For this review, take the finished solid that the model builds, in its own axes (mm). A direction names the side the tool comes from. Coordinates: 2 decimals unless noted, no trailing zeros. Use one line per item in the form item = value.
```python
from build123d import *

# Parameters (mm, degrees)
F0_W     = 400
F0_H     = 50
F1_DEPTH = 300
F3_DEPTH = 600.001


with BuildPart() as f1:
    # F0 (on Right) → F1 (new body, symmetric)
    with BuildSketch(Plane.YZ):
        with Locations((0, -25)):
            Rectangle(F0_W, F0_H)
    extrude(amount=F1_DEPTH, both=True)

    # F2 (on face) → F3 (cut, through all)
    with BuildSketch(Plane.YZ.offset(300)):
        Polygon((-162, 0), (-174, 0), (-174, -6), (-176.5, -6), (-176.5, -14), (-159.5, -14), (-159.5, -6), (-162, -6), align=None)
        Polygon((-128.5, -6), (-128.5, -14), (-111.5, -14), (-111.5, -6), (-114, -6), (-114, 0), (-126, 0), (-126, -6), align=None)
        Polygon((-80.5, -6), (-80.5, -14), (-63.5, -14), (-63.5, -6), (-66, -6), (-66, 0), (-78, 0), (-78, -6), align=None)
        Polygon((-32.5, -6), (-32.5, -14), (-15.5, -14), (-15.5, -6), (-18, -6), (-18, 0), (-30, 0), (-30, -6), align=None)
        Polygon((15.5, -6), (15.5, -14), (32.5, -14), (32.5, -6), (30, -6), (30, 0), (18, 0), (18, -6), align=None)
        Polygon((63.5, -6), (63.5, -14), (80.5, -14), (80.5, -6), (78, -6), (78, 0), (66, 0), (66, -6), align=None)
        Polygon((111.5, -6), (111.5, -14), (128.5, -14), (128.5, -6), (126, -6), (126, 0), (114, 0), (114, -6), align=None)
        Polygon((159.5, -6), (159.5, -14), (176.5, -14), (176.5, -6), (174, -6), (174, 0), (162, 0), (162, -6), align=None)
    extrude(amount=-F3_DEPTH, mode=Mode.SUBTRACT)


solid = f1.part
```
1. For pin 1 Ø2 at (x, y) = (149.5, 146) entering from +Z; pin 2 Ø8.5 at (x, y) = (40.5, 71) entering from +Z, all flat-tipped, find the tip position at first contact; note any pin that passes through.
Computed values:
pin_1 = 0
pin_2 = -14
2. Wall thickness on line 1 along Z through (x, y) = (266, 161); line 2 along Z through (x, y) = (51, 29): over which ranges is each line inside the solid? List them lowest first. Write a range as from..to.
Computed values:
line_1 = -50..-14, -6..0
line_2 = -50..-14
3. Draft analysis for pull direction Z (two halves, no side actions). For faces 3 (the face through (4, 72, -14)), 4 (the face through (4, -200, -25)), 5 (the face through (4, 96, 0)), state which applies: +Z half, -Z half, draft (parallel to the pull), parting line (faces both ways), or undercut.
Computed values:
face_3 = undercut
face_4 = draft
face_5 = +Z half
4. Tool access review of faces 1 (the face through (4, -168, -14)), 2 (the face through (4, -144, 0)): name each direction out of +Z, -Z, +X, -X, +Y, -Y from which nothing blocks a thin tool from reaching the whole face with its end or side.
Computed values:
face_1 = +X, -X
face_2 = +Z, +X, -X, +Y, -Y
